from build123d import *

# Parameters (mm, degrees)
SKETCH_1_W               = 62
SKETCH_1_H               = 62
EXTRUDE_1_DEPTH          = 10
SKETCH_2_W               = 61
SKETCH_2_H               = 61
EXTRUDE_2_DEPTH          = 60
SKETCH_3_W               = 62
SKETCH_3_H               = 62
EXTRUDE_3_DEPTH          = 38
CUT_EXTRUDE_START        = -98
SKETCH_4_W               = 14.732123786
SKETCH_4_H               = 13.996978426
CUT_EXTRUDE_1_DEPTH      = 98
FILLET_1_R               = 4
FILLET_3_R               = 4
SKETCH_5_R               = 4
EXTRUDE_4_DEPTH          = 20
PATTERN_CIRCULAR_4_COUNT = 4
FILLET_4_R               = 4
FILLET_5_R               = 4
CHAMFER_1_SIZE           = 5
SKETCH_6_R               = 25
EXTRUDE_5_DEPTH          = 3
SKETCH_7_R               = 3
CUT_EXTRUDE_2_DEPTH      = 12
PATTERN_CIRCULAR_5_COUNT = 4
CHAMFER_2_SIZE           = 0.5
SKETCH_8_W               = 26
SKETCH_8_H               = 20
EXTRUDE_6_DEPTH          = 14
SKETCH_9_R               = 3.083920488
EXTRUDE_7_DEPTH          = 14
FILLET_START             = 9
FILLET_6_DEPTH           = 21
FILLET_START_2           = 10
FILLET_6_2_DEPTH         = 20
PATTERN_LINEAR_2_COUNT   = 2
PATTERN_LINEAR_2_PITCH   = 60
FILLET_7_R               = 4


with BuildPart() as part:
    # 草图1 → 凸台-拉伸1 (new body)
    with BuildSketch(Plane.XY):
        Rectangle(SKETCH_1_W, SKETCH_1_H)
    extrude(amount=EXTRUDE_1_DEPTH)

    # 草图2 → 凸台-拉伸2 (add)
    with BuildSketch(Plane.XY.offset(10)):
        Rectangle(SKETCH_2_W, SKETCH_2_H)
    extrude(amount=EXTRUDE_2_DEPTH)

    # 草图3 → 凸台-拉伸3 (add)
    with BuildSketch(Plane.XY.offset(70)):
        Rectangle(SKETCH_3_W, SKETCH_3_H)
    extrude(amount=EXTRUDE_3_DEPTH)

    # 草图4 → 切除-拉伸1 (cut)
    with BuildSketch(Plane.XY.offset(108).offset(CUT_EXTRUDE_START)):
        with Locations((-28.366061893, 27.998489213)):
            Rectangle(SKETCH_4_W, SKETCH_4_H)
    cut_extrude_1 = extrude(amount=CUT_EXTRUDE_1_DEPTH, mode=Mode.SUBTRACT)

    # 圆角1
    fillet_1_edges = [part.edges().sort_by_distance(p)[0] for p in [
        (-21, 21, 59),
    ]]
    fillet(fillet_1_edges, radius=FILLET_1_R)

    # 圆角3
    fillet_3_edges = [part.edges().sort_by_distance(p)[0] for p in [
        (-31, 21, 89),
        (-21, 31, 89),
    ]]
    fillet(fillet_3_edges, radius=FILLET_3_R)

    # 草图5 → 凸台-拉伸4 (add)
    with BuildSketch(Plane(origin=(0, 0, 0), x_dir=(-1, 0, 0), z_dir=(0, 0, -1))):
        Circle(SKETCH_5_R)
    extrude(amount=EXTRUDE_4_DEPTH)

    # 阵列(圆周)4: 切除-拉伸1 ×4 about axis
    pattern_circular_4_axis = Axis((0, 0, 0), (0, 0, 1))
    for i in range(1, PATTERN_CIRCULAR_4_COUNT):
        add(cut_extrude_1.rotate(pattern_circular_4_axis, i * 360 / PATTERN_CIRCULAR_4_COUNT), mode=Mode.SUBTRACT)

    # 圆角4
    fillet_4_edges = [part.edges().sort_by_distance(p)[0] for p in [
        (-21, -21, 59),
        (21, -21, 59),
        (21, 21, 59),
    ]]
    fillet(fillet_4_edges, radius=FILLET_4_R)

    # 圆角5
    fillet_5_edges = [part.edges().sort_by_distance(p)[0] for p in [
        (-31, -21, 89),
        (-21, -31, 89),
        (21, -31, 89),
        (31, -21, 89),
        (31, 21, 89),
        (21, 31, 89),
    ]]
    fillet(fillet_5_edges, radius=FILLET_5_R)

    # 倒角1
    chamfer_1_edges = [part.edges().sort_by_distance(p)[0] for p in [
        (31, -31, 5),
        (-31, -31, 5),
        (-31, 31, 5),
        (31, 31, 5),
    ]]
    chamfer(chamfer_1_edges, length=CHAMFER_1_SIZE)

    # 草图6 → 凸台-拉伸5 (add)
    with BuildSketch(Plane(origin=(0, 0, 0), x_dir=(-1, 0, 0), z_dir=(0, 0, -1))):
        Circle(SKETCH_6_R)
    extrude(amount=EXTRUDE_5_DEPTH)

    # 草图7 → 切除-拉伸2 (cut)
    with BuildSketch(Plane(origin=(0, 0, 0), x_dir=(-1, 0, 0), z_dir=(0, 0, -1))):
        with Locations((24.748737342, 24.748737342)):
            Circle(SKETCH_7_R)
    cut_extrude_2 = extrude(amount=-CUT_EXTRUDE_2_DEPTH, mode=Mode.SUBTRACT)

    # 阵列(圆周)5: 切除-拉伸2 ×4 about axis
    pattern_circular_5_axis = Axis((0, 0, 0), (0, 0, 1))
    for i in range(1, PATTERN_CIRCULAR_5_COUNT):
        add(cut_extrude_2.rotate(pattern_circular_5_axis, i * 360 / PATTERN_CIRCULAR_5_COUNT), mode=Mode.SUBTRACT)

    # 倒角2
    chamfer_2_edges = [part.edges().sort_by_distance(p)[0] for p in [
        (25, 0, -3),
        (4, 0, -20),
    ]]
    chamfer(chamfer_2_edges, length=CHAMFER_2_SIZE)

    # 草图8 → 凸台-拉伸6 (add)
    with BuildSketch(Plane(origin=(0, 30.5, 0), x_dir=(1, 0, 0), z_dir=(0, 1, 0))):
        with Locations((0, -20)):
            Rectangle(SKETCH_8_W, SKETCH_8_H)
    extrude_6 = extrude(amount=EXTRUDE_6_DEPTH)

    # 草图9 → 凸台-拉伸7 (add)
    with BuildSketch(Plane.XY.offset(30)):
        with Locations(Location((0, 39.131165124, 0), (0, 0, 180))):
            Circle(SKETCH_9_R)
    extrude_7 = extrude(amount=EXTRUDE_7_DEPTH)

    # 圆角6: read off the stored shape, not the designer's step
    # 圆角6 outline → 圆角6 (cut)
    with BuildSketch(Plane.XY.offset(FILLET_START)):
        with BuildLine():
            ThreePointArc((9, 44.5), (11.828427125, 43.328427125), (13, 40.5))
            Line((13, 40.5), (13, 44.5))
            Line((13, 44.5), (9, 44.5))
        make_face()
        with BuildLine():
            ThreePointArc((-13, 40.5), (-11.828427125, 43.328427125), (-9, 44.5))
            Line((-9, 44.5), (-13, 44.5))
            Line((-13, 44.5), (-13, 40.5))
        make_face()
    extrude(amount=FILLET_6_DEPTH, mode=Mode.SUBTRACT)

    # Fillet 6 2 outline → Fillet 6 2 (add)
    with BuildSketch(Plane.XY.offset(FILLET_START_2)):
        with BuildLine():
            ThreePointArc((17, 30.5), (14.171572875, 31.671572875), (13, 34.5))
            Line((13, 34.5), (13, 30.5))
            Line((13, 30.5), (17, 30.5))
        make_face()
        with BuildLine():
            Line((-17, 30.5), (-13, 30.5))
            Line((-13, 30.5), (-13, 34.5))
            ThreePointArc((-13, 34.5), (-14.171572875, 31.671572875), (-17, 30.5))
        make_face()
    extrude(amount=FILLET_6_2_DEPTH)

    # 阵列(线性)2: 凸台-拉伸6, 凸台-拉伸7 ×2
    with Locations(*[(0, 0, i * PATTERN_LINEAR_2_PITCH) for i in range(1, PATTERN_LINEAR_2_COUNT)]):
        add(extrude_6)
        add(extrude_7)

    # 圆角7
    fillet_7_edges = [part.edges().sort_by_distance(p)[0] for p in [
        (13, 31, 80),
        (-13, 31, 80),
    ]]
    fillet(fillet_7_edges, radius=FILLET_7_R - 0.0001)  # a hair under: the kernel refuses the full size
    fillet_7_2_edges = [part.edges().sort_by_distance(p)[0] for p in [
        (13, 44.5, 80),
        (-13, 44.5, 80),
    ]]
    fillet(fillet_7_2_edges, radius=FILLET_7_R)


solid = part.part
Could you check a few things on this model? Use its own coordinates, in mm. A direction names the side the tool comes from. Give positions to 0.01 mm unless a question says otherwise; leave off trailing zeros. Order: outer loops, then holes, each group sorted by start corner. A loop starts at its lowest first (then second) coordinate and runs counter-clockwise, first axis right, second up.
1. For faces 1 (the flat face through (13, 38, 80)), 2 (the cylindrical face through (-20.3, 29.26, 59.69)), 3 (the cylindrical face through (20.3, 29.26, 58.31)), which set-ups out of +Z, -Z, +X, -X, +Y, -Y let a thin tool reach every point of the face, with its end or its side?
2. Suppose I cut it at A-A (z = 92). List the corners of the cut face in (x, y) for me, plus the area to 3 significant figures.
3. Suppose I cut it at C-C (z = 67). List the corners of the cut face in (x, y) for me.
4. Suppose I cut it at B-B (y = 0). List the corners of the cut face in (x, z) for me, plus the area to 3 significant figures.
5. I need wall thicknesses on L1, parallel to Z at x = -13.5, y = -7.5; L2, parallel to X at y = -22, z = 6; L3, parallel to Y at x = 10.5, z = 32. Which ranges of each line are inside material? Lowest first, please.
6. We'd pull the mould along Y, two halves only. Please class faces 4 (the flat face through (0, -31, 5)), 5 (the cylindrical face through (-27.52, 23.6, 4.93)), 6 (the flat face through (-5, 0, -3)), 7 (the cylindrical face through (14.203, 31.641, 19.86)): pulls with the +Y half, pulls with the -Y half, needs draft (parallel to the pull), parting line crosses it, or undercut.
7. Will these pins go through, and if not, where does the flat tip stop? P1, Ø2, axis at x = 24.5, z = 93, coming from the -Y side; P2, Ø7, axis at x = -1.5, y = 38.5, coming from the +Z side; P3, Ø2, axis at y = -13, z = 34.5, coming from the -X side.
Solved:
1. face 1: +Z, -Z, +X, +Y
1. face 2: +Z, -X, +Y
1. face 3: +Z, +X, +Y
2. outline: (-31, -17) arc R4 ccw to (-27, -21) - (-25, -21) arc R4 cw to (-21, -25) - (-21, -27) arc R4 ccw to (-17, -31) - (17, -31) arc R4 ccw to (21, -27) - (21, -25) arc R4 cw to (25, -21) - (27, -21) arc R4 ccw to (31, -17) - (31, 17) arc R4 ccw to (27, 21) - (25, 21) arc R4 cw to (21, 25) - (21, 27) arc R4 ccw to (17, 31) - (-17, 31) arc R4 ccw to (-21, 27) - (-21, 25) arc R4 cw to (-25, 21) - (-27, 21) arc R4 ccw to (-31, 17) - close; circle Ø6.17 at (0, 39.13)
2. area: 3,460 mm2
3. outline: (-30.5, -18.94) arc R4 ccw to (-27, -21) - (-25, -21) arc R4 cw to (-21, -25) - (-21, -27) arc R4 ccw to (-18.94, -30.5) - (18.94, -30.5) arc R4 ccw to (21, -27) - (21, -25) arc R4 cw to (25, -21) - (27, -21) arc R4 ccw to (30.5, -18.94) - (30.5, 18.94) arc R4 ccw to (27, 21) - (25, 21) arc R4 cw to (21, 25) - (21, 27) arc R4 ccw to (18.94, 30.5) - (-18.94, 30.5) arc R4 ccw to (-21, 27) - (-21, 25) arc R4 cw to (-25, 21) - (-27, 21) arc R4 ccw to (-30.5, 18.94) - close
4. outline: (-31, 0) - (-25, 0) - (-25, -2.5) - (-24.5, -3) - (-4, -3) - (-4, -19.5) - (-3.5, -20) - (3.5, -20) - (4, -19.5) - (4, -3) - (24.5, -3) - (25, -2.5) - (25, 0) - (31, 0) - (31, 10) - (30.5, 10) - (30.5, 70) - (31, 70) - (31, 108) - (-31, 108) - (-31, 70) - (-30.5, 70) - (-30.5, 10) - (-31, 10) - close
4. area: 6,920 mm2
5. L1: z = -3 to 108
5. L2: x = -31 to -25.95, -23.55 to 23.55, 25.95 to 31
5. L3: y = -30.5 to 30.5
6. face 4: pulls with the -Y half
6. face 5: undercut
6. face 6: needs draft
6. face 7: pulls with the +Y half
7. P1: stops at y = -21.29
7. P2: stops at z = 104
7. P3: stops at x = -30.5
